Autodesk Fusion 360 part; units mm, degrees
sketch "Sketch1" plane through (0, 0, 0) normal (0, 0, 1) x (1, 0, 0)
  line L0 (0, 6) -> (0, 1)
  line L1 (1, 0) -> (10, 0)
  line L2 (10, 0) -> (10, 1)
  line L3 (10, 1) -> (5, 1)
  line L4 (5, 1) -> (1, 6)
  line L5 (1, 6) -> (0, 6)
  arc A0 (0, 1) -> (1, 0) centre (1, 1) ccw
  dimension "d1" = 6
  dimension "d2" = 10
  dimension "d3" = 1
  dimension "d4" = 5
  dimension "d5" = 1
  dimension "d6" = 1
extrude "Extrude1" add sketch "Sketch1" along normal blind 5
sketch "Sketch2" plane through (3.5366, 2.8293, 0) normal (0.7809, 0.6247, 0) x (0, 0, -1)
  line L0 (0, -2.3426) -> (0, 4.0605)
  line L1 (0, 4.0605) -> (-5, 4.0605)
  line L2 (-5, 4.0605) -> (-5, -2.3426)
  line L3 (-5, -2.3426) -> (0, -2.3426)
  circle A0 centre (-2.5, 0.8605) radius 1.4
  dimension "d9" = 2.8
  dimension "d10" = 3.2
  dimension "d11" = 2.5
extrude "Extrude2" cut sketch "Sketch2" against normal blind 1 contours A0
fillet "Fillet1" radius 0.2 1 edges at (1.9019, 3.2718, 3.8053)
fillet "Fillet2" radius 1 1 edges at (10, 0.5, 5)
fillet "Fillet3" radius 1 1 edges at (10, 0.5, 0)
sketch "Sketch3" plane through (0, 1, 0) normal (0, 1, 0) x (-1, 0, 0)
  arc A0 (-10, 1) -> (-9, 0) centre (-9, 1) ccw
  line L0 (-9, 0) -> (-5, 0)
  line L1 (-5, 0) -> (-5, 5)
  line L2 (-5, 5) -> (-9, 5)
  arc A1 (-9, 5) -> (-10, 4) centre (-9, 4) ccw
  line L3 (-10, 4) -> (-10, 1)
  circle A2 centre (-9, 1) radius 0.5
  circle A3 centre (-9, 4) radius 0.5
  dimension "d17" = 1
  dimension "d18" = 1
  dimension "d19" = 4
extrude "Extrude3" cut sketch "Sketch3" against normal through all contours A2 | A3
Design review of the part built by this model. Coordinates are the model's own, in mm. A direction names the side the tool comes from. Round coordinates to 2 decimals unless told otherwise and drop trailing zeros. Write each loop counter-clockwise with the first axis right and the second up, starting at its lowest first coordinate (ties: lowest second). Pieces come first, ordered by that corner, then holes. Notation, with made-up numbers: M 51.5,38 L 92.5,38 A24 cw 92.5,60 Z; hole C 29.25,-35.75 d6. An arc over 180 degrees is marked long. One line per item, written item: value. Start each with the question number.
1. Take a section at B-B on y = 1.65. State the section outline as (x, z) points, then the cut area to 3 significant figures.
2. Clearance check with a flat-ended pin moving along its axis: P1, Ø2, axis at x = 6.5, z = 3.5, coming from the -Y side. State where the tip first meets the part, or that it passes through.
3. To check wall thickness, follow probe 1 along Z at (x, y) = (9, 0.65); probe 2 along Y at (x, z) = (7, 1.35); probe 3 along Y at (x, z) = (3, 4.25). State the ranges of each line that lie inside material, in increasing order. Write a range as from..to.
4. Draft analysis for pull direction X (two halves, no side actions). For faces 4 (the face through (8.538, 0.507, 0.808)), 5 (the face through (0, 4, 2)), 6 (the face through (2, 2, 5)), 7 (the face through (9.715, 0.507, 0.301)), state which applies: pulls with the +X half, pulls with the -X half, needs draft (parallel to the pull), parting line crosses it, or undercut.
5. For faces 1 (the face through (2.2, 2.9, 2.5)), 2 (the face through (10, 0.5, 2.5)), 3 (the face through (8, 1, 2)), list the 3-axis set-ups (+Z, -Z, +X, -X, +Y, -Y) from which the entire face can be reached by the end or side of a thin tool; tool diameter is ignored.
6. Take a section at A-A on z = 0.65. State the section outline as (x, y) points, then the cut area to 3 significant figures.
7. Take a section at C-C on z = 4.65. State the section outline as (x, y) points, then the cut area to 3 significant figures.
8. Take a section at D-D on x = 6.75. State the section outline as (y, z) points.
Computed:
1. outline: M 0,0 L 4.48,0 L 4.48,5 L 0,5 Z
1. area: 22.4 mm²
2. P1: stops at y = 0
3. probe 1: z = 0..0.5, 1.5..3.5, 4.5..5
3. probe 2: y = 0..1
3. probe 3: y = 0..3.5
4. face 4: undercut
4. face 5: pulls with the -X half
4. face 6: needs draft
4. face 7: pulls with the +X half
5. face 1: none
5. face 2: +Z, -Z, +X, +Y, -Y
5. face 3: +Z, -Z, +X, +Y
6. outline: M 0,1 A1 ccw 1,0 L 8.64,0 L 8.64,1 L 5,1 L 1,6 L 0,6 Z; M 9.36,0 L 9.94,0 L 9.94,1 L 9.36,1 Z
6. area: 24.0 mm²
7. outline: M 0,1 A1 ccw 1,0 L 9.76,0 L 9.76,1 L 5,1 L 1,6 L 0,6 Z
7. area: 24.5 mm²
8. outline: M 0,0 L 1,0 L 1,5 L 0,5 Z
